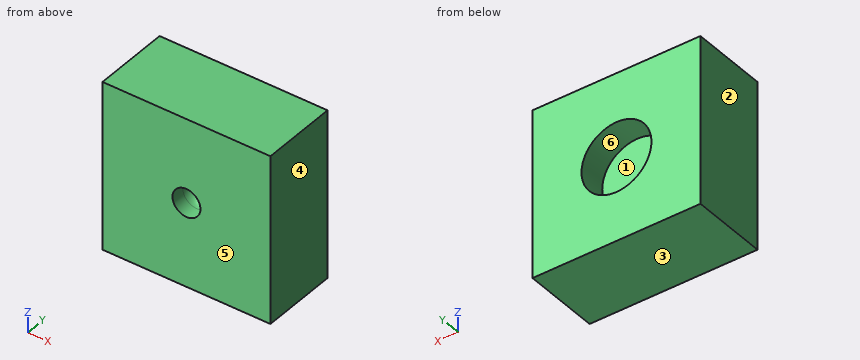
from build123d import *

# Parameters (mm, degrees)
SKETCH1_W           = 12
SKETCH1_H           = 12
BOSS_EXTRUDE1_DEPTH = 5.5
SKETCH2_R           = 2.5
CUT_EXTRUDE1_DEPTH  = 2
SKETCH4_R           = 1
CUT_EXTRUDE3_DEPTH  = 2
FILLET2_R           = 1


with BuildPart() as part:
    # Sketch1 → Boss-Extrude1 (new body)
    with BuildSketch(Plane(origin=(0, 0, 0), x_dir=(1, 0, 0), z_dir=(0, 1, 0))):
        Rectangle(SKETCH1_W, SKETCH1_H)
    extrude(amount=BOSS_EXTRUDE1_DEPTH)

    # Sketch2 → Cut-Extrude1 (cut)
    with BuildSketch(Plane(origin=(0, 5.5, 0), x_dir=(1, 0, 0), z_dir=(0, 1, 0))):
        Circle(SKETCH2_R)
    extrude(amount=-CUT_EXTRUDE1_DEPTH, mode=Mode.SUBTRACT)

    # Sketch4 → Cut-Extrude3 (cut)
    with BuildSketch(Plane.XZ):
        Circle(SKETCH4_R)
    extrude(amount=-CUT_EXTRUDE3_DEPTH, mode=Mode.SUBTRACT)

    # Fillet2
    fillet2_edges = [part.edges().sort_by_distance(p)[0] for p in [
        (-1, 2, 0),
    ]]
    fillet(fillet2_edges, radius=FILLET2_R)


solid = part.part
Model file for the job. Use its own axes, mm. Face numbers are marked on the shaded views. A direction names the side the tool comes from. Give positions to 0.01 mm unless a question says otherwise; leave off trailing zeros. Order: outer loops, then holes, each group sorted by start corner. A loop starts at its lowest first (then second) coordinate and runs counter-clockwise, first axis right, second up. Notation, with made-up numbers: (-12, -13) - (41, -13) arc R29 cw to (41, 18) - close; hole circle Ø8 at (5, -23). An arc over 180 degrees is marked (long way). One line per item, written item: value.
Item 1: Tool access for the marked faces 5 and 6: list every direction of +Z, -Z, +X, -X, +Y, -Y with a clear straight run to the whole face (end or side of a thin tool).
Response values:
face 5: +Z, -Z, +X, -X, -Y
face 6: +Y
Item 2: Pin check, flat tips, straight feed: pin 1 Ø1.5 at (x, z) = (1, 1) entering from +Y; pin 2 Ø1.6 at (x, z) = (0, 0) entering from -Y; pin 3 Ø6 at (x, z) = (0, 0) entering from -Y. Stop position of each tip, or through.
Response values:
pin 1: y = 3.5
pin 2: y = 1.6
pin 3: y = 0
Item 3: Two-plate mould, pull along X, no slides. Class the marked faces 1, 2, 3 and 4: released by +X, released by -X, zero draft, split by the parting line, or undercut.
Response values:
face 1: undercut
face 2: released by -X
face 3: zero draft
face 4: released by +X
Item 4: Wall check: line 1 (X direction, y = 4.85, z = 0); line 2 (Z direction, x = 0, y = 0.6). Give the ranges that are in metal, low to high.
Response values:
line 1: -6 to -2.5, 2.5 to 6
line 2: -6 to -1, 1 to 6
Item 5: Slice it at C-C (z = 0). List the corners of the cut face in (x, y).
Response values:
outline: (-6, 0) - (-1, 0) - (-1, 1) arc R1 cw to (1, 1) - (1, 0) - (6, 0) - (6, 5.5) - (2.5, 5.5) - (2.5, 3.5) - (-2.5, 3.5) - (-2.5, 5.5) - (-6, 5.5) - close
Item 6: Slice it at A-A (y = 4.85). List the corners of the cut face in (x, z).
Response values:
outline: (-6, -6) - (6, -6) - (6, 6) - (-6, 6) - close; hole circle Ø5 at (0, 0)
Item 7: Slice it at B-B (x = 0). List the corners of the cut face in (y, z), then the cut area to 3 significant figures.
Response values:
outline: (0, -6) - (5.5, -6) - (5.5, -2.5) - (3.5, -2.5) - (3.5, 2.5) - (5.5, 2.5) - (5.5, 6) - (0, 6) - (0, 1) - (1, 1) arc R1 cw to (1, -1) - (0, -1) - close
area: 52.4 mm2
Item 8: Slice it at D-D (y = 0.6). List the corners of the cut face in (x, z), then the cut area to 3 significant figures.
Response values:
outline: (-6, -6) - (6, -6) - (6, 6) - (-6, 6) - close; hole circle Ø2 at (0, 0)
area: 141 mm2
